Read the model definition and answer for the solid it produces. Units are mm, in the model's axes. Face numbers are marked on the shaded views. A direction names the side the tool comes from. Coordinates: 2 decimals unless noted, no trailing zeros. Write item = value, one per line.
from build123d import *

# Parameters (mm, degrees)
SKETCH1_W           = 9
SKETCH1_H           = 25
SKETCH1_W_2         = 0.83
SKETCH1_W_3         = 9.32
BOSS_EXTRUDE1_DEPTH = 10


with BuildPart() as part:
    # Sketch1 → Boss-Extrude1 (new body)
    with BuildSketch(Plane(origin=(0, 0, 0), x_dir=(0, 0, -1), z_dir=(1, 0, 0))):
        with BuildLine():
            Line((23.938201687, 1), (39.9, 1))
            Line((39.9, 1), (39.9, 28))
            Line((39.9, 28), (-39.9, 28))
            Line((-39.9, 28), (-39.9, 1))
            Line((-39.9, 1), (-23.938201687, 1))
            ThreePointArc((-23.938201687, 1), (0, 15.75), (23.938201687, 1))
        make_face()
        with Locations((-34.4, 14.5)):
            Rectangle(SKETCH1_W, SKETCH1_H, mode=Mode.SUBTRACT)
        with Locations((-28.685, 14.5)):
            Rectangle(SKETCH1_W_2, SKETCH1_H, mode=Mode.SUBTRACT)
        with Locations((-27.055, 14.5)):
            Rectangle(SKETCH1_W_2, SKETCH1_H, mode=Mode.SUBTRACT)
        with Locations((-25.425, 14.5)):
            Rectangle(SKETCH1_W_2, SKETCH1_H, mode=Mode.SUBTRACT)
        with BuildLine():
            Line((-24.21, 27), (-23.38, 27))
            Line((-23.38, 27), (-23.38, 3.990465418))
            ThreePointArc((-23.38, 3.990465418), (-23.80494512, 3.308432638), (-24.21, 2.614402658))
            Line((-24.21, 2.614402658), (-24.21, 27))
        make_face(mode=Mode.SUBTRACT)
        with BuildLine():
            Line((-22.58, 27), (-21.75, 27))
            Line((-21.75, 27), (-21.75, 6.264083863))
            ThreePointArc((-21.75, 6.264083863), (-22.171789507, 5.720562008), (-22.58, 5.166769099))
            Line((-22.58, 5.166769099), (-22.58, 27))
        make_face(mode=Mode.SUBTRACT)
        with BuildLine():
            Line((-20.95, 27), (-20.12, 27))
            Line((-20.12, 27), (-20.12, 8.133993328))
            ThreePointArc((-20.12, 8.133993328), (-20.540040569, 7.683572361), (-20.95, 7.223956879))
            Line((-20.95, 7.223956879), (-20.95, 27))
        make_face(mode=Mode.SUBTRACT)
        with BuildLine():
            Line((-19.32, 27), (-18.49, 27))
            Line((-18.49, 27), (-18.49, 9.709573695))
            ThreePointArc((-18.49, 9.709573695), (-18.908921242, 9.328731498), (-19.32, 8.939437211))
            Line((-19.32, 8.939437211), (-19.32, 27))
        make_face(mode=Mode.SUBTRACT)
        with BuildLine():
            Line((-17.69, 27), (-16.86, 27))
            Line((-16.86, 27), (-16.86, 11.053854867))
            ThreePointArc((-16.86, 11.053854867), (-17.278137213, 10.72856686), (-17.69, 10.39537013))
            Line((-17.69, 10.39537013), (-17.69, 27))
        make_face(mode=Mode.SUBTRACT)
        with BuildLine():
            Line((-16.06, 27), (-15.23, 27))
            Line((-15.23, 27), (-15.23, 12.206979598))
            ThreePointArc((-15.23, 12.206979598), (-15.647552225, 11.928122407), (-16.06, 11.641769433))
            Line((-16.06, 11.641769433), (-16.06, 27))
        make_face(mode=Mode.SUBTRACT)
        with BuildLine():
            Line((-14.43, 27), (-13.6, 27))
            Line((-13.6, 27), (-13.6, 13.196236821))
            ThreePointArc((-13.6, 13.196236821), (-14.017094411, 12.957520994), (-14.43, 12.711630836))
            Line((-14.43, 12.711630836), (-14.43, 27))
        make_face(mode=Mode.SUBTRACT)
        with BuildLine():
            Line((-12.8, 27), (-11.97, 27))
            Line((-11.97, 27), (-11.97, 14.041016321))
            ThreePointArc((-11.97, 14.041016321), (-12.386722167, 13.83793109), (-12.8, 13.627925359))
            Line((-12.8, 13.627925359), (-12.8, 27))
        make_face(mode=Mode.SUBTRACT)
        with BuildLine():
            Line((-11.17, 27), (-10.34, 27))
            Line((-10.34, 27), (-10.34, 14.755511039))
            ThreePointArc((-10.34, 14.755511039), (-10.756409627, 14.584735262), (-11.17, 14.40724062))
            Line((-11.17, 14.40724062), (-11.17, 27))
        make_face(mode=Mode.SUBTRACT)
        with BuildLine():
            Line((-9.54, 27), (-8.71, 27))
            Line((-8.71, 27), (-8.71, 15.350301135))
            ThreePointArc((-8.71, 15.350301135), (-9.126139757, 15.209352108), (-9.54, 15.061844056))
            Line((-9.54, 15.061844056), (-9.54, 27))
        make_face(mode=Mode.SUBTRACT)
        with BuildLine():
            Line((-7.91, 27), (-7.08, 27))
            Line((-7.08, 27), (-7.08, 15.833333127))
            ThreePointArc((-7.08, 15.833333127), (-7.495900758, 15.720346875), (-7.91, 15.600926813))
            Line((-7.91, 15.600926813), (-7.91, 27))
        make_face(mode=Mode.SUBTRACT)
        with BuildLine():
            Line((-6.28, 27), (-5.45, 27))
            Line((-5.45, 27), (-5.45, 16.210548417))
            ThreePointArc((-5.45, 16.210548417), (-5.865684067, 16.124137529), (-6.28, 16.031388443))
            Line((-6.28, 16.031388443), (-6.28, 27))
        make_face(mode=Mode.SUBTRACT)
        with BuildLine():
            Line((-4.65, 27), (-3.82, 27))
            Line((-3.82, 27), (-3.82, 16.486296047))
            ThreePointArc((-3.82, 16.486296047), (-4.235483175, 16.425455998), (-4.65, 16.358347269))
            Line((-4.65, 16.358347269), (-4.65, 27))
        make_face(mode=Mode.SUBTRACT)
        with BuildLine():
            Line((-3.02, 27), (-2.19, 27))
            Line((-2.19, 27), (-2.19, 16.663604962))
            ThreePointArc((-2.19, 16.663604962), (-2.605292879, 16.62765252), (-3.02, 16.585477199))
            Line((-3.02, 16.585477199), (-3.02, 27))
        make_face(mode=Mode.SUBTRACT)
        with BuildLine():
            Line((-1.39, 27), (-0.56, 27))
            Line((-0.56, 27), (-0.56, 16.74435914))
            ThreePointArc((-0.56, 16.74435914), (-0.97510879, 16.732893349), (-1.39, 16.715228254))
            Line((-1.39, 16.715228254), (-1.39, 27))
        make_face(mode=Mode.SUBTRACT)
        with BuildLine():
            Line((0.24, 27), (1.07, 27))
            Line((1.07, 27), (1.07, 16.729400641))
            ThreePointArc((1.07, 16.729400641), (0.655073035, 16.74228093), (0.24, 16.748964009))
            Line((0.24, 16.748964009), (0.24, 27))
        make_face(mode=Mode.SUBTRACT)
        with BuildLine():
            Line((1.87, 27), (2.7, 27))
            Line((2.7, 27), (2.7, 16.618574231))
            ThreePointArc((2.7, 16.618574231), (2.285256378, 16.655912786), (1.87, 16.687034809))
            Line((1.87, 16.687034809), (1.87, 27))
        make_face(mode=Mode.SUBTRACT)
        with BuildLine():
            Line((3.5, 27), (4.33, 27))
            Line((4.33, 27), (4.33, 16.410719219))
            ThreePointArc((4.33, 16.410719219), (3.915445127, 16.472886648), (3.5, 16.528796203))
            Line((3.5, 16.528796203), (3.5, 27))
        make_face(mode=Mode.SUBTRACT)
        with BuildLine():
            Line((5.13, 27), (5.96, 27))
            Line((5.96, 27), (5.96, 16.103607495))
            ThreePointArc((5.96, 16.103607495), (5.54564356, 16.191252495), (5.13, 16.272574915))
            Line((5.13, 16.272574915), (5.13, 27))
        make_face(mode=Mode.SUBTRACT)
        with BuildLine():
            Line((6.76, 27), (7.59, 27))
            Line((7.59, 27), (7.59, 15.693819847))
            ThreePointArc((7.59, 15.693819847), (7.175856686, 15.807905369), (6.76, 15.915578058))
            Line((6.76, 15.915578058), (6.76, 27))
        make_face(mode=Mode.SUBTRACT)
        with BuildLine():
            Line((8.39, 27), (9.22, 27))
            Line((9.22, 27), (9.22, 15.176543806))
            ThreePointArc((9.22, 15.176543806), (8.806090708, 15.3184047), (8.39, 15.453733699))
            Line((8.39, 15.453733699), (8.39, 27))
        make_face(mode=Mode.SUBTRACT)
        with BuildLine():
            Line((10.02, 27), (10.85, 27))
            Line((10.85, 27), (10.85, 14.545263234))
            ThreePointArc((10.85, 14.545263234), (10.43635371, 14.71669403), (10.02, 14.881440377))
            Line((10.02, 14.881440377), (10.02, 27))
        make_face(mode=Mode.SUBTRACT)
        with BuildLine():
            Line((11.65, 27), (12.48, 27))
            Line((12.48, 27), (12.48, 13.791288211))
            ThreePointArc((12.48, 13.791288211), (12.066656732, 13.994675988), (11.65, 14.191186581))
            Line((11.65, 14.191186581), (11.65, 27))
        make_face(mode=Mode.SUBTRACT)
        with BuildLine():
            Line((13.28, 27), (14.11, 27))
            Line((14.11, 27), (14.11, 12.903035298))
            ThreePointArc((14.11, 12.903035298), (13.697015562, 13.141563916), (13.28, 13.372972792))
            Line((13.28, 13.372972792), (13.28, 27))
        make_face(mode=Mode.SUBTRACT)
        with BuildLine():
            Line((14.91, 27), (15.74, 27))
            Line((15.74, 27), (15.74, 11.864894719))
            ThreePointArc((15.74, 11.864894719), (15.327453929, 12.142868646), (14.91, 12.413416205))
            Line((14.91, 12.413416205), (14.91, 27))
        make_face(mode=Mode.SUBTRACT)
        with BuildLine():
            Line((16.54, 27), (17.37, 27))
            Line((17.37, 27), (17.37, 10.655370303))
            ThreePointArc((17.37, 10.655370303), (16.958009538, 10.978751951), (16.54, 11.294314713))
            Line((16.54, 11.294314713), (16.54, 27))
        make_face(mode=Mode.SUBTRACT)
        with BuildLine():
            Line((18.17, 27), (19, 27))
            Line((19, 27), (19, 9.24384143))
            ThreePointArc((19, 9.24384143), (18.588746526, 9.621199835), (18.17, 9.990225759))
            Line((18.17, 9.990225759), (18.17, 27))
        make_face(mode=Mode.SUBTRACT)
        with BuildLine():
            Line((19.8, 27), (20.63, 27))
            Line((20.63, 27), (20.63, 7.584460014))
            ThreePointArc((20.63, 7.584460014), (20.219784013, 8.028792794), (19.8, 8.464097468))
            Line((19.8, 8.464097468), (19.8, 27))
        make_face(mode=Mode.SUBTRACT)
        with BuildLine():
            Line((21.43, 27), (22.26, 27))
            Line((22.26, 27), (22.26, 5.603299973))
            ThreePointArc((22.26, 5.603299973), (21.851371771, 6.135969619), (21.43, 6.658616547))
            Line((21.43, 6.658616547), (21.43, 27))
        make_face(mode=Mode.SUBTRACT)
        with BuildLine():
            Line((23.06, 27), (23.89, 27))
            Line((23.89, 27), (23.89, 3.166465806))
            ThreePointArc((23.89, 3.166465806), (23.484138497, 3.827339784), (23.06, 4.47663518))
            Line((23.06, 4.47663518), (23.06, 27))
        make_face(mode=Mode.SUBTRACT)
        with Locations((25.105, 14.5)):
            Rectangle(SKETCH1_W_2, SKETCH1_H, mode=Mode.SUBTRACT)
        with Locations((26.735, 14.5)):
            Rectangle(SKETCH1_W_2, SKETCH1_H, mode=Mode.SUBTRACT)
        with Locations((28.365, 14.5)):
            Rectangle(SKETCH1_W_2, SKETCH1_H, mode=Mode.SUBTRACT)
        with Locations((34.24, 14.5)):
            Rectangle(SKETCH1_W_3, SKETCH1_H, mode=Mode.SUBTRACT)
    extrude(amount=BOSS_EXTRUDE1_DEPTH)


solid = part.part
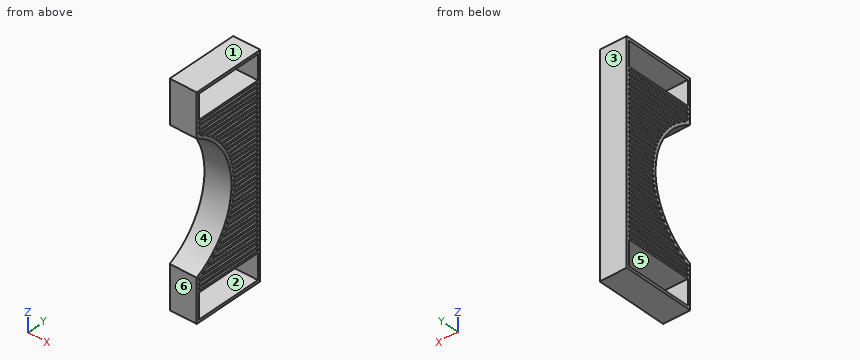
1) Determine the mould class of the marked faces 1, 2, 3 and 4 for opening direction Z: pulls with the +Z half, pulls with the -Z half, needs draft (parallel to the pull), parting line crosses it, or undercut.
Returned:
face_1 = pulls with the +Z half
face_2 = undercut
face_3 = needs draft
face_4 = undercut
2) For the marked faces 5 and 6, determine the directions among +Z, -Z, +X, -X, +Y, -Y from which every point of the face is accessible in a straight line to the end or side of a thin tool.
Returned:
face_5 = +X, -X
face_6 = +Z, -Z, +X, -X, -Y
3) A flat-ended cylindrical pin translates along its axis: pin 1 Ø0.9 at (x, z) = (6.5, 2.5) entering from -Y. Find the tip coordinate at first contact, or state that the pin passes through.
Returned:
pin_1 = 15.59
4) Straight lines are drawn through the part: line 1 along Y through (x, z) = (0.75, 6); line 2 along Y through (x, z) = (5.25, 31); line 3 along Y through (x, z) = (5.25, -14.5). For each, find the intervals that lie inside material, in ascending order. Write a range as from..to.
Returned:
line_1 = 15.07..16.09, 27..28
line_2 = 1..2, 27..28
line_3 = 11.49..28
5) The part is cut by section A-A (y = 17.5). Count the separate pieces of the cut face and the enclosed holes in it, and give its area (3 significant figures).
Returned:
separate_pieces = 39
enclosed_holes = 0
area = 316 mm^2
